Geometry check sheet. Reference: the model listing, model coordinates, mm. Face numbers are marked on the shaded views. A direction names the side the tool comes from. Round coordinates to 2 decimals unless told otherwise and drop trailing zeros. Order: outer loops, then holes, each group sorted by start corner. A loop starts at its lowest first (then second) coordinate and runs counter-clockwise, first axis right, second up. Notation, with made-up numbers: (26.5, -1) - (55.5, -1) arc R10 cw to (55.5, 14) - close; hole circle Ø6 at (32.5, -10.75). An arc over 180 degrees is marked (long way). Return JSON: item names as keys, results as strings. Group by question number.
Q1. Sectioned sample at A-A, the plane y = 8.5. Record the cut outline in (x, z).
Q2. Sectioned sample at B-B, the plane z = 1.5. Record the cut outline in (x, y).
Q3. Gauge pin test, flat ends, axial feed: pin 1 Ø16 at (x, y) = (0.5, 10.5) entering from -Z; pin 2 Ø5 at (x, z) = (-5, 1) entering from -Y; pin 3 Ø6 at (x, z) = (3, -1.5) entering from +Y. Record the tip position at first contact, or that the pin passes through.
Q4. Sectioned sample at C-C, the plane y = 32. Record the cut outline in (x, z), then the cut area to 3 significant figures.
Q5. Tool access check on the marked faces 1, 2, 3 and 4. Record the directions out of +Z, -Z, +X, -X, +Y, -Y that give a thin tool (end or side, any length) a straight path to the whole face; none if there is none.
Q6. Sectioned sample at D-D, the plane x = -7.25. Record the cut outline in (y, z), then the cut area to 3 significant figures.
Q7. Draft check along X on the marked faces 5, 6 and 7. Enter one of: pulls with the +X half, pulls with the -X half, needs draft (parallel to the pull), parting line crosses it, or undercut.
Q8. Material ranges on line 1 along Z through (x, y) = (0, 5.5); line 2 along X through (y, z) = (34.5, -3.5); line 3 along Z through (x, y) = (11.5, 16), recorded low to high.
```python
from build123d import *

# Parameters (mm, degrees)
RESSALTO_EXTRUS_O1_DEPTH = 15
CORTE_EXTRUS_O1_DEPTH    = 10


with BuildPart() as part:
    # Esboço1 → Ressalto-extrusão1 (new body, symmetric)
    with BuildSketch(Plane(origin=(0, 0, 0), x_dir=(0, 0, -1), z_dir=(1, 0, 0))):
        Polygon((-20, 0), (-20, 40), (20, 40), (20, 0), (5, 0), (5, 20), (-5, 20), (-5, 0), align=None)
    extrude(amount=RESSALTO_EXTRUS_O1_DEPTH, both=True)

    # Esboço2 → Corte-extrusão1 (cut, symmetric)
    with BuildSketch(Plane(origin=(0, 0, 0), x_dir=(0, 0, -1), z_dir=(1, 0, 0))):
        Polygon((-10, 0), (-10, 30), (10, 30), (10, 0), (20, 0), (20, 40), (-20, 40), (-20, 0), align=None)
    extrude(amount=CORTE_EXTRUS_O1_DEPTH, both=True, mode=Mode.SUBTRACT)


solid = part.part
```
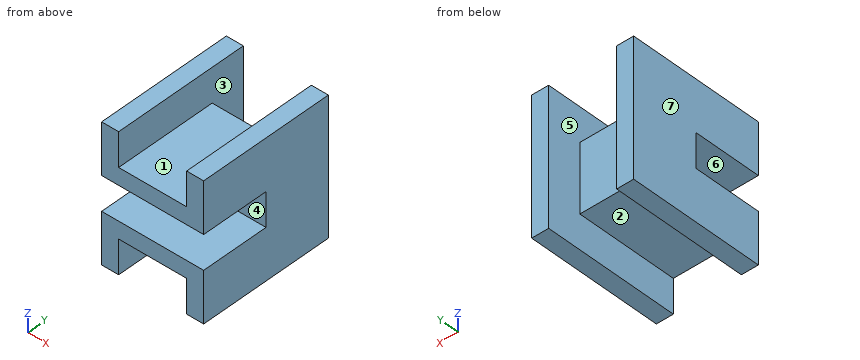
Reply:
{
 "1": {"outline": "(-15, -20) - (-10, -20) - (-10, -10) - (10, -10) - (10, -20) - (15, -20) - (15, -5) - (-15, -5) - close; (-15, 5) - (15, 5) - (15, 20) - (10, 20) - (10, 10) - (-10, 10) - (-10, 20) - (-15, 20) - close"},
 "2": {"outline": "(-15, 20) - (15, 20) - (15, 40) - (10, 40) - (10, 30) - (-10, 30) - (-10, 40) - (-15, 40) - close"},
 "3": {"pin 1": "z = -10", "pin 2": "y = 20", "pin 3": "y = 30"},
 "4": {"outline": "(-15, -20) - (-10, -20) - (-10, 20) - (-15, 20) - close; (10, -20) - (15, -20) - (15, 20) - (10, 20) - close", "area": "400 mm^2"},
 "5": {"face 1": "+Z, +Y, -Y", "face 2": "-Z, +Y, -Y", "face 3": "+Y", "face 4": "+X, -X, -Y"},
 "6": {"outline": "(0, -10) - (30, -10) - (30, 10) - (0, 10) - (0, 5) - (20, 5) - (20, -5) - (0, -5) - close", "area": "400 mm^2"},
 "7": {"face 5": "undercut", "face 6": "needs draft", "face 7": "pulls with the -X half"},
 "8": {"line 1": "-10 to -5, 5 to 10", "line 2": "-15 to -10, 10 to 15", "line 3": "-20 to -5, 5 to 20"}
}
